Build history of the part. All positions in model axes, mm. Face numbers are marked on the shaded views. A direction names the side the tool comes from. Give positions to 0.01 mm unless a question says otherwise; leave off trailing zeros. Order: outer loops, then holes, each group sorted by start corner. A loop starts at its lowest first (then second) coordinate and runs counter-clockwise, first axis right, second up. Notation, with made-up numbers: (34, -19.5) - (53, -19.5) arc R7 ccw to (53, -14.5) - close; hole circle Ø2 at (-7, 65.25). An arc over 180 degrees is marked (long way). Use a Markdown table: item, result. Add a question column.
(1) Wall check: line 1 (Z direction, x = 19, y = 14); line 2 (Z direction, x = -21, y = 18.5); line 3 (Z direction, x = -18, y = -11). Give the ranges that are in metal, low to high.
(2) Slice it at B-B (z = 8). Write the cut outline in (x, y), then the cut area to 3 significant figures.
(3) Mould opens along Z. For the marked faces 3, 4 and 5 say: +Z half, -Z half, draft (parallel to the pull), parting line (faces both ways), or undercut.
(4) Which spindle directions (+Z, -Z, +X, -X, +Y, -Y) get a long thin tool onto all of the face, cutting with end or side? Do the marked faces 1 and 2. Say none if no direction does.
(5) Slice it at A-A (x = 18). Write the cut outline in (y, z), then the cut area to 3 significant figures.
(6) Slice it at D-D (x = -7.5). Write the cut outline in (y, z), then the cut area to 3 significant figures.
(7) Flat gauge pins, fed straight in: pin 1 (2 mm diameter, centred on x = -8, z = -22.5, fed in from -Y); pin 2 (3 mm diameter, centred on y = -5.5, z = 16, fed in from -X); pin 3 (15 mm diameter, centred on y = 0, z = 0, fed in from -X); pin 4 (6 mm diameter, centred on x = -21.5, z = -21.5, fed in from +Y). Where does each tip first touch, or does it go through?
from build123d import *

# Parameters (mm, degrees)
CROQUIS1_R                                           = 32.7
CROQUIS1_R_2                                         = 21
SALIENTE_EXTRUIR1_DEPTH                              = 24.25
SALIENTE_EXTRUIR2_START                              = 3.5
CROQUIS2_R                                           = 32.7
CROQUIS2_R_2                                         = 12.5
SALIENTE_EXTRUIR2_DEPTH                              = 3.5
CROQUIS3_R                                           = 32.7
SALIENTE_EXTRUIR3_DEPTH                              = 5
CROQUIS4_R                                           = 3.5
CORTAR_EXTRUIR1_DEPTH                                = 6
REFRENTADO_PARA_TORNILLO_TAP_N_CON_CABEZ_D           = 3.4
REFRENTADO_PARA_TORNILLO_TAP_N_CON_CABEZ_CSINK_D     = 6.72
REFRENTADO_PARA_TORNILLO_TAP_N_CON_CABEZ_CSINK_ANGLE = 90
TALADRO_DE_MARGEN_PARA_M31_D                         = 3.4
TALADRO_DE_MARGEN_PARA_M31_DEPTH                     = 15
TALADRO_DE_MARGEN_PARA_M31_TIP                       = 1.021463052


with BuildPart() as part:
    # Croquis1 → Saliente-Extruir1 (new, symmetric)
    with BuildSketch(Plane(origin=(0, 0, 0), x_dir=(0, 0, -1), z_dir=(1, 0, 0))):
        with Locations(Location((0, 0, 0), (0, 0, 180))):
            Circle(CROQUIS1_R)
        with Locations(Location((0, 0, 0), (0, 0, 180))):
            Circle(CROQUIS1_R_2, mode=Mode.SUBTRACT)
    extrude(amount=SALIENTE_EXTRUIR1_DEPTH, both=True)

    # Croquis2 → Saliente-Extruir2 (add)
    with BuildSketch(Plane(origin=(24.25, 0, 0), x_dir=(0, 0, -1), z_dir=(1, 0, 0)).offset(SALIENTE_EXTRUIR2_START)):
        with Locations(Location((0, 0, 0), (0, 0, 180))):
            Circle(CROQUIS2_R)
        Circle(CROQUIS2_R_2, mode=Mode.SUBTRACT)
    extrude(amount=-SALIENTE_EXTRUIR2_DEPTH)

    # Croquis3 → Saliente-Extruir3 (add)
    with BuildSketch(Plane.ZY.offset(24.25)):
        Circle(CROQUIS3_R)
        with BuildLine():
            Line((-18, 21), (18, 21))
            ThreePointArc((18, 21), (20.121320344, 20.121320344), (21, 18))
            Line((21, 18), (21, -18))
            ThreePointArc((21, -18), (20.121320344, -20.121320344), (18, -21))
            Line((18, -21), (-18, -21))
            ThreePointArc((-18, -21), (-20.121320344, -20.121320344), (-21, -18))
            Line((-21, -18), (-21, 18))
            ThreePointArc((-21, 18), (-20.121320344, 20.121320344), (-18, 21))
        make_face(mode=Mode.SUBTRACT)
    extrude(amount=SALIENTE_EXTRUIR3_DEPTH)

    # Croquis4 → Cortar-Extruir1 (cut)
    with BuildSketch(Plane.ZY.offset(24.25)):
        with Locations((15.5, 15.5)):
            Circle(CROQUIS4_R)
        with Locations((-15.5, 15.5)):
            Circle(CROQUIS4_R)
        with Locations((-15.5, -15.5)):
            Circle(CROQUIS4_R)
        with Locations((15.5, -15.5)):
            Circle(CROQUIS4_R)
    extrude(amount=-CORTAR_EXTRUIR1_DEPTH, mode=Mode.SUBTRACT)

    # Refrentado para tornillo tapón con cabeza plana de clavija de M32 (through all)
    with Locations(Plane(origin=(27.75, 0, 0), x_dir=(0, 0, -1), z_dir=(1, 0, 0))):
        with Locations((12.375, 12.375), (-12.375, -12.375), (-12.375, 12.375), (12.375, -12.375)):
            CounterSinkHole(REFRENTADO_PARA_TORNILLO_TAP_N_CON_CABEZ_D / 2, REFRENTADO_PARA_TORNILLO_TAP_N_CON_CABEZ_CSINK_D / 2, counter_sink_angle=REFRENTADO_PARA_TORNILLO_TAP_N_CON_CABEZ_CSINK_ANGLE)

    # Taladro de margen para M31
    with Locations(Plane(origin=(27.75, 0, 0), x_dir=(0, 0, -1), z_dir=(1, 0, 0))):
        with Locations((0, 29), (25.11473671, 14.5), (25.11473671, -14.5), (0, -29), (-25.11473671, -14.5), (-25.11473671, 14.5)):
            Hole(TALADRO_DE_MARGEN_PARA_M31_D / 2, depth=TALADRO_DE_MARGEN_PARA_M31_DEPTH)
            with Locations((0, 0, -(TALADRO_DE_MARGEN_PARA_M31_DEPTH + TALADRO_DE_MARGEN_PARA_M31_TIP / 2))):  # 118° drill point
                Cone(0, TALADRO_DE_MARGEN_PARA_M31_D / 2, TALADRO_DE_MARGEN_PARA_M31_TIP, mode=Mode.SUBTRACT)


solid = part.part
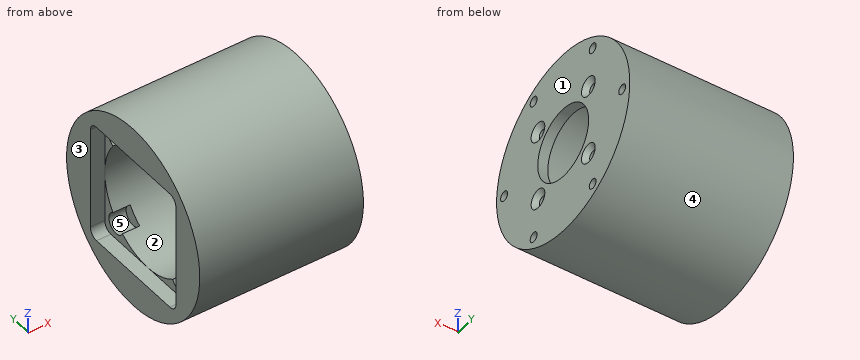
Solution:
| question | item | result |
|---|---|---|
| 1 | line 1 | -29.55 to -26.74, -23.49 to -15.65, 15.65 to 23.49, 26.74 to 29.55 |
| 1 | line 2 | -26.96 to -17.3, -13.7 to -9.94, 9.94 to 13.7, 17.3 to 26.96 |
| 1 | line 3 | -30.79 to -17.89, 17.89 to 30.79 |
| 2 | outline | (-29.25, -31.71) - (27.75, -31.71) - (27.75, -9.6) - (24.25, -9.6) - (24.25, -19.42) - (-24.25, -19.42) - (-24.25, -21) - (-29.25, -21) - close; (-29.25, 21) - (-24.25, 21) - (-24.25, 19.42) - (24.25, 19.42) - (24.25, 9.6) - (27.75, 9.6) - (27.75, 31.71) - (-29.25, 31.71) - close |
| 2 | area | 1,450 mm2 |
| 3 | face 3 | draft |
| 3 | face 4 | parting line |
| 3 | face 5 | undercut |
| 4 | face 1 | +Z, -Z, +X, +Y, -Y |
| 4 | face 2 | -X |
| 5 | outline | circle Ø65.4 at (0, 0); hole circle Ø3.4 at (-29, 0); hole circle Ø42 at (0, 0); hole circle Ø3.4 at (-14.5, -25.11); hole circle Ø3.4 at (-14.5, 25.11); hole circle Ø3.4 at (14.5, -25.11); hole circle Ø3.4 at (14.5, 25.11); hole circle Ø3.4 at (29, 0) |
| 5 | area | 1,920 mm2 |
| 6 | outline | circle Ø65.4 at (0, 0); hole circle Ø42 at (0, 0) |
| 6 | area | 1,970 mm2 |
| 7 | pin 1 | y = -24.64 |
| 7 | pin 2 | x = 24.25 |
| 7 | pin 3 | through |
| 7 | pin 4 | y = 26.96 |
